Check sheet for the modelled part. Datum: model origin and axes. Units: mm. A direction names the side the tool comes from. Round coordinates to 2 decimals unless told otherwise and drop trailing zeros. Write each loop counter-clockwise with the first axis right and the second up, starting at its lowest first coordinate (ties: lowest second). Pieces come first, ordered by that corner, then holes. Notation, with made-up numbers: M -32,-14.5 L -18,-14.5 A22 cw -18,-1.5 Z; hole C -24.75,11 d1. An arc over 180 degrees is marked long. One line per item, written item: value.
from build123d import *

# Parameters (mm, degrees)
SKETCH1_W           = 121.6
SKETCH1_H           = 72
BOSS_EXTRUDE1_DEPTH = 3
CUT_EXTRUDE1_REACH  = 5
SKETCH4_W           = 42
SKETCH4_H           = 22
SKETCH6_W           = 3
SKETCH6_H           = 10.285714
SKETCH6_H_2         = 10.316450419
SKETCH6_H_3         = 10.26857
SKETCH6_H_4         = 10.29
CUT_EXTRUDE2_DEPTH  = 4
SKETCH7_W           = 17.37142857
SKETCH7_H           = 3
BOSS_EXTRUDE2_DEPTH = 3


with BuildPart() as part:
    # Sketch1 → Boss-Extrude1 (new body)
    with BuildSketch(Plane.XY):
        with Locations((60.8, 36)):
            Rectangle(SKETCH1_W, SKETCH1_H)
    extrude(amount=BOSS_EXTRUDE1_DEPTH)

    # Sketch4 → Cut-Extrude1 (cut, up to next)
    with BuildSketch(Plane.XY.offset(3), mode=Mode.PRIVATE) as cut_extrude1_sk1:
        with Locations((94.6, 58)):
            Rectangle(SKETCH4_W, SKETCH4_H)
    cut_extrude1_tool1 = extrude(cut_extrude1_sk1.sketch, amount=-CUT_EXTRUDE1_REACH, mode=Mode.PRIVATE) & part.part
    add(cut_extrude1_tool1.solids().sort_by_distance((94.6, 58, 3))[0], mode=Mode.SUBTRACT)

    # Sketch6 → Cut-Extrude2 (cut, through all)
    with BuildSketch(Plane.XY.offset(3)):
        with Locations((120.1, 56.571428714)):
            Rectangle(SKETCH6_W, SKETCH6_H)
        with Locations((120.1, 36.015368924)):
            Rectangle(SKETCH6_W, SKETCH6_H_2)
        with Locations((120.1, 15.428572714)):
            Rectangle(SKETCH6_W, SKETCH6_H)
        with Locations((1.5, 15.420000714)):
            Rectangle(SKETCH6_W, SKETCH6_H_3)
        with Locations((1.5, 35.989285714)):
            Rectangle(SKETCH6_W, SKETCH6_H_4)
        with Locations((1.5, 56.569285714)):
            Rectangle(SKETCH6_W, SKETCH6_H_4)
    extrude(amount=-CUT_EXTRUDE2_DEPTH, mode=Mode.SUBTRACT)

    # Sketch7 → Boss-Extrude2 (add)
    with BuildSketch(Plane.XY.offset(3)):
        with Locations((95.542857144, -1.5)):
            Rectangle(SKETCH7_W, SKETCH7_H)
        with Locations((60.800000004, -1.5)):
            Rectangle(SKETCH7_W, SKETCH7_H)
        with Locations((26.057142864, -1.5)):
            Rectangle(SKETCH7_W, SKETCH7_H)
    extrude(amount=-BOSS_EXTRUDE2_DEPTH)


solid = part.part
Q1. Scan lines: line 1 (Y direction, x = 102, z = 0.7); line 2 (X direction, y = 54.5, z = 2.5); line 3 (X direction, y = 49.5, z = 1.1). Record each from-to range of solid material in increasing order. Write a range as [from, to].
Completed:
line 1: [-3, 47], [69, 72]
line 2: [3, 73.6], [115.6, 118.6]
line 3: [0, 73.6], [115.6, 121.6]
Q2. Sectioned sample at A-A on x = 113.5. Enter the section's corners in (y, z).
Completed:
outline: M 0,0 L 47,0 L 47,3 L 0,3 Z; M 69,0 L 72,0 L 72,3 L 69,3 Z
Q3. Depth check by flat-ended pin: P1, Ø1.5, axis at x = 119.5, z = 1, coming from the -Y side. Enter the tip coordinate at first touch or a pass-through.
Completed:
P1: y = 0
Q4. Sectioned sample at C-C on y = 37.5. Enter the section's corners in (x, z), and give its area (3 significant figures).
Completed:
outline: M 3,0 L 118.6,0 L 118.6,3 L 3,3 Z
area: 347 mm^2
Q5. Sectioned sample at B-B on y = 49. Enter the section's corners in (x, z), and give its area (3 significant figures).
Completed:
outline: M 0,0 L 73.6,0 L 73.6,3 L 0,3 Z; M 115.6,0 L 121.6,0 L 121.6,3 L 115.6,3 Z
area: 239 mm^2
Q6. Sectioned sample at D-D on x = 48. Enter the section's corners in (y, z), and give its area (3 significant figures).
Completed:
outline: M 0,0 L 72,0 L 72,3 L 0,3 Z
area: 216 mm^2
Q7. Draft check along X on faces 4 (the flat face through (118.6, 56, 2)), 5 (the flat face through (86.857, -2, 2)), 6 (the flat face through (115.6, 58, 2)), 7 (the flat face through (0, 26, 1)). Enter one of: pulls with the +X half, pulls with the -X half, needs draft (parallel to the pull), parting line crosses it, or undercut.
Completed:
face 4: pulls with the +X half
face 5: undercut
face 6: undercut
face 7: pulls with the -X half
Q8. Access from +Z, -Z, +X, -X, +Y, -Y to the whole of each face (thin tool, end or side, straight path). Record for faces 1 (the flat face through (78, 0, 1)), 2 (the flat face through (1, 30.844, 2)), 3 (the flat face through (120, 10.286, 2)).
Completed:
face 1: +Z, -Z, -Y
face 2: +Z, -Z, -X
face 3: +Z, -Z, +X
